Autodesk Fusion 360 part; units mm, degrees
sketch "Sketch1" plane through (0, 0, 0) normal (0, 0, 1) x (1, 0, 0)
  circle A0 centre (0, 0) radius 19.25
  circle A1 centre (0, 0) radius 13.725
  line L0 (0, 0) -> (4.5, 0)
  line L1 (4.5, 0) -> (4.5, 19.25)
  line L2 (4.5, 19.25) -> (0, 19.25)
  line L3 (0, 19.25) -> (0, 0)
  line L4 (0, 0) -> (-4.5, 0)
  line L5 (-4.5, 0) -> (-4.5, 19.25)
  line L6 (-4.5, 19.25) -> (0, 19.25)
  line L7 (0, 19.25) -> (0, 0)
  line L8 (4.5, 19.25) -> (-4.5, 19.25)
  line L9 (-4.5, 19.25) -> (-4.5, 26.25)
  line L10 (-4.5, 26.25) -> (4.5, 26.25)
  line L11 (4.5, 26.25) -> (4.5, 19.25)
  line L12 (0, 19.25) -> (2, 19.25)
  line L13 (2, 19.25) -> (2, 23)
  line L14 (2, 23) -> (0, 23)
  line L15 (0, 23) -> (0, 19.25)
  line L16 (0, 19.25) -> (-2, 19.25)
  line L17 (-2, 19.25) -> (-2, 23)
  line L18 (-2, 23) -> (0, 23)
  line L19 (0, 23) -> (0, 19.25)
  dimension "d1" = 38.5
  dimension "d2" = 27.45
  dimension "d3" = 4.5
  dimension "d4" = 19.25
  dimension "d5" = 4.5
  dimension "d6" = 19.25
  dimension "d7" = 7
extrude "Extrude1" add sketch "Sketch1" along normal blind 2 contours A0 A1 L1 L5 | A0 A1 L1 L3 L7 | A0 L1 L2 L8 L12 | A0 L5 L6 L8 L16 | A0 A1 L3 L5 L7 | L2 L6 L8 L9 L10 L11 L13 L14 L17 L18
fillet "Fillet1" radius 1 1 edges at (-2, 23, 1)
fillet "Fillet2" radius 1 1 edges at (2, 23, 1)
fillet "Fillet3" radius 2.5 1 edges at (-4.5, 26.25, 1)
fillet "Fillet4" radius 2.5 1 edges at (4.5, 26.25, 1)
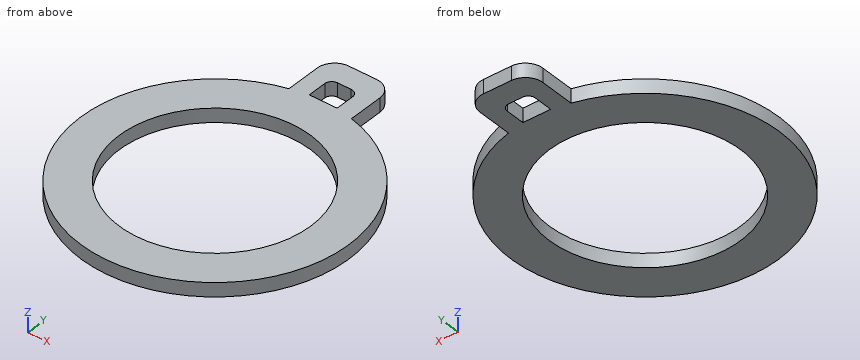
Work out the finished part from the listing and answer in its coordinate system (mm). Give positions to 0.01 mm unless a question says otherwise; leave off trailing zeros. Loops run counter-clockwise (first coordinate to the right, second up) from the corner with the lowest first, then second, coordinate; pieces in that order, holes last. Notation, with made-up numbers: M 58.5,81.25 L 84.5,81.25 A15 cw 84.5,95.25 Z; hole C 49,52.25 d7. An arc over 180 degrees is marked long. One line per item, written item: value. Start each with the question number.
1. Find the intervals of material crossed by probe 1 along Y at (x, z) = (0, 0.8) (3 decimals); probe 2 along X at (y, z) = (0, 1.35) (3 decimals); probe 3 along X at (y, z) = (21, 0.7), in increasing order.
2. Find section C-C (z = 1.4). Give the vertices of the cut face in (x, y) (3 decimals), and give its area (3 significant figures).
3. Each of these flat-tipped pins is pushed along its axis until it touches: P1, Ø1, axis at y = 20, z = 0.5, coming from the +X side; P2, Ø1, axis at y = 21.5, z = 1.5, coming from the -X side. Where does it stop, or does it pass through?
4. Find section A-A (x = 0). Give the vertices of the cut face in (y, z) (3 decimals).
5. Find section D-D (x = 11). Give the vertices of the cut face in (y, z), and give its area (3 significant figures).
6. Find section B-B (y = 0). Give the vertices of the cut face in (x, z) (3 decimals), and give its area (3 significant figures).
Reported:
1. probe 1: y = -19.25 to -13.725, 13.725 to 19.25, 23 to 26.25
1. probe 2: x = -19.25 to -13.725, 13.725 to 19.25
1. probe 3: x = -4.5 to -2, 2 to 4.5
2. outline: M -4.5,18.717 A19.25 ccw long 4.5,18.717 L 4.5,23.75 A2.5 ccw 2,26.25 L -2,26.25 A2.5 ccw -4.5,23.75 Z; hole C 0,0 d27.45; hole M -2,19.25 L 2,19.25 L 2,22 A1 ccw 1,23 L -1,23 A1 ccw -2,22 Z
2. area: 620 mm²
3. P1: stops at x = 4.5
3. P2: stops at x = -4.5
4. outline: M -19.25,0 L -13.725,0 L -13.725,2 L -19.25,2 Z; M 13.725,0 L 19.25,0 L 19.25,2 L 13.725,2 Z; M 23,0 L 26.25,0 L 26.25,2 L 23,2 Z
5. outline: M -15.8,0 L -8.21,0 L -8.21,2 L -15.8,2 Z; M 8.21,0 L 15.8,0 L 15.8,2 L 8.21,2 Z
5. area: 30.4 mm²
6. outline: M -19.25,0 L -13.725,0 L -13.725,2 L -19.25,2 Z; M 13.725,0 L 19.25,0 L 19.25,2 L 13.725,2 Z
6. area: 22.1 mm²
